```python
from build123d import *

# Parameters (mm, degrees)
SKETCH2_W                = 10
SKETCH2_H                = 10.5
BOSS_EXTRUDE1_DEPTH      = 2
SKETCH3_W                = 12.5
SKETCH3_H                = 14.5
BOSS_EXTRUDE2_DEPTH      = 3.5
SKETCH4_W                = 14.6
SKETCH4_H                = 14.5
BOSS_EXTRUDE3_DEPTH      = 3.5
SKETCH5_W                = 12.5
SKETCH5_H                = 14.5
BOSS_EXTRUDE4_DEPTH      = 4.3
BOSS_EXTRUDE5_DEPTH      = 2.3
SKETCH8_W                = 12.1
SKETCH8_H                = 11.1
CUT_EXTRUDE1_DEPTH       = 13
SKETCH10_W               = 3.5
SKETCH10_H               = 0.7
CUT_EXTRUDE6_DEPTH       = 4
FILLET1_R                = 1
CUT_EXTRUDE9_DEPTH       = 18.994790913
CUT_EXTRUDE9_DEPTH_BACK  = 18.994790913
SKETCH15_W               = 3
SKETCH15_H               = 5
BOSS_EXTRUDE6_DEPTH      = 0.7
FILLET5_R                = 0.5
FILLET3_R                = 1
FILLET4_R                = 1
CUT_EXTRUDE10_DEPTH      = 20.550255917
CUT_EXTRUDE10_DEPTH_BACK = 2
SKETCH14_W               = 4.56
SKETCH14_H               = 10
CHAMFER4_SIZE            = 1.5


with BuildPart() as part:
    # Sketch2 → Boss-Extrude1 (new body)
    with BuildSketch(Plane.YZ):
        Rectangle(SKETCH2_W, SKETCH2_H)
    extrude(amount=BOSS_EXTRUDE1_DEPTH)

    # Sketch3 → Boss-Extrude2 (add)
    with BuildSketch(Plane(origin=(0, 0, 0), x_dir=(0, -1, 0), z_dir=(-1, 0, 0))):
        with Locations((0, 2)):
            Rectangle(SKETCH3_W, SKETCH3_H)
    extrude(amount=BOSS_EXTRUDE2_DEPTH)

    # Sketch4 → Boss-Extrude3 (add)
    with BuildSketch(Plane(origin=(-3.5, 0, 0), x_dir=(0, -1, 0), z_dir=(-1, 0, 0))):
        with Locations((0, 2)):
            Rectangle(SKETCH4_W, SKETCH4_H)
    extrude(amount=BOSS_EXTRUDE3_DEPTH)

    # Sketch5 → Boss-Extrude4 (add)
    with BuildSketch(Plane(origin=(-7, 0, 0), x_dir=(0, -1, 0), z_dir=(-1, 0, 0))):
        with Locations((0, 2)):
            Rectangle(SKETCH5_W, SKETCH5_H)
    extrude(amount=BOSS_EXTRUDE4_DEPTH)

    # Sketch6 → Boss-Extrude5 (add)
    with BuildSketch(Plane(origin=(-11.3, 0, 0), x_dir=(0, -1, 0), z_dir=(-1, 0, 0))):
        Polygon((6.25, -5.25), (7.3, -5.25), (7.3, 9.25), (6.25, 9.25), (-6.25, 9.25), (-7.3, 9.25), (-7.3, -5.25), (-6.25, -5.25), align=None)
    extrude(amount=BOSS_EXTRUDE5_DEPTH)

    # Sketch8 → Cut-Extrude1 (cut)
    with BuildSketch(Plane.XY.offset(9.25)):
        with Locations((-7.55, 0)):
            Rectangle(SKETCH8_W, SKETCH8_H)
    extrude(amount=-CUT_EXTRUDE1_DEPTH, mode=Mode.SUBTRACT)

    # Sketch10 → Cut-Extrude6 (cut)
    with BuildSketch(Plane.XY.offset(9.25)):
        with Locations((-1.75, 5.9)):
            Rectangle(SKETCH10_W, SKETCH10_H)
        with Locations((-1.75, -5.9)):
            Rectangle(SKETCH10_W, SKETCH10_H)
    extrude(amount=-CUT_EXTRUDE6_DEPTH, mode=Mode.SUBTRACT)

    # Fillet1
    fillet1_edges = [part.edges().sort_by_distance(p)[0] for p in [
        (-13.6, -5.55, 2.75),
        (-13.6, 5.55, 2.75),
    ]]
    fillet(fillet1_edges, radius=FILLET1_R)

    # Sketch13 → Cut-Extrude9 (cut, two sides: drawn at the far end of the back side and taken through both)
    with BuildSketch(Plane(origin=(0, 0, 0), x_dir=(0, 0, -1), z_dir=(1, 0, 0)).offset(-CUT_EXTRUDE9_DEPTH_BACK)):
        with BuildLine():
            Line((-2.045, 0.01001), (-2.045, -3.17999))
            ThreePointArc((-2.045, -3.17999), (-1.611518036, -4.226508036), (-0.565, -4.65999))
            Line((-0.565, -4.65999), (0.035, -4.65999))
            ThreePointArc((0.035, -4.65999), (1.081518036, -4.226508036), (1.515, -3.17999))
            Line((1.515, -3.17999), (1.515, 0.01001))
            Line((1.515, 0.01001), (1.515, 3.20001))
            ThreePointArc((1.515, 3.20001), (1.081518036, 4.246528036), (0.035, 4.68001))
            Line((0.035, 4.68001), (-0.565, 4.68001))
            ThreePointArc((-0.565, 4.68001), (-1.611518036, 4.246528036), (-2.045, 3.20001))
            Line((-2.045, 3.20001), (-2.045, 0.01001))
        make_face()
    extrude(amount=CUT_EXTRUDE9_DEPTH + CUT_EXTRUDE9_DEPTH_BACK, mode=Mode.SUBTRACT)

    # Sketch15 → Boss-Extrude6 (add)
    with BuildSketch(Plane.XY.offset(-3.75)):
        with BuildLine():
            Line((-13.6, 6.55), (-13.6, -6.55))
            ThreePointArc((-13.6, -6.55), (-13.307106781, -5.842893219), (-12.6, -5.55))
            Line((-12.6, -5.55), (-1.5, -5.55))
            Line((-1.5, -5.55), (-1.5, 5.55))
            Line((-1.5, 5.55), (-12.6, 5.55))
            ThreePointArc((-12.6, 5.55), (-13.307106781, 5.842893219), (-13.6, 6.55))
        make_face()
        with Locations((-4.5, 0)):
            Rectangle(SKETCH15_W, SKETCH15_H, mode=Mode.SUBTRACT)
    extrude(amount=BOSS_EXTRUDE6_DEPTH)

    # Fillet5
    fillet5_edges = [part.edges().sort_by_distance(p)[0] for p in [
        (-3, 2.5, -3.4),
        (-6, 2.5, -3.4),
        (-6, -2.5, -3.4),
        (-3, -2.5, -3.4),
    ]]
    fillet(fillet5_edges, radius=FILLET5_R)

    # Fillet3
    fillet3_edges = [part.edges().sort_by_distance(p)[0] for p in [
        (-1.5, -5.55, 1.1),
        (-1.5, 5.55, 1.1),
    ]]
    fillet(fillet3_edges, radius=FILLET3_R)

    # Fillet4
    fillet4_edges = [part.edges().sort_by_distance(p)[0] for p in [
        (-13.307106781, 5.842893219, -3.05),
        (-13.307106781, -5.842893219, -3.05),
        (-7.55, -5.55, -3.05),
        (-7.55, 5.55, -3.05),
        (-1.5, 0, -3.05),
        (-1.792893219, -5.257106781, -3.05),
        (-1.792893219, 5.257106781, -3.05),
    ]]
    fillet(fillet4_edges, radius=FILLET4_R)

    # Sketch14 → Cut-Extrude10 (cut, two sides: drawn at the far end of the back side and taken through both)
    with BuildSketch(Plane(origin=(2, 0, 0), x_dir=(0, 0, -1), z_dir=(1, 0, 0)).offset(-CUT_EXTRUDE10_DEPTH_BACK)):
        with Locations((-0.265, 0)):
            Rectangle(SKETCH14_W, SKETCH14_H)
    extrude(amount=CUT_EXTRUDE10_DEPTH + CUT_EXTRUDE10_DEPTH_BACK, mode=Mode.SUBTRACT)

    # Chamfer4
    chamfer4_edges = [part.edges().sort_by_distance(p)[0] for p in [
        (2, 0, 2.545),
        (2, 0, -2.015),
    ]]
    chamfer(chamfer4_edges, length=CHAMFER4_SIZE)


solid = part.part
```
Verification items for the finished model (mm, model axes). A direction names the side the tool comes from. Give positions to 0.01 mm unless a question says otherwise; leave off trailing zeros. Order: outer loops, then holes, each group sorted by start corner. A loop starts at its lowest first (then second) coordinate and runs counter-clockwise, first axis right, second up. Notation, with made-up numbers: M 10.25,42 L 46.25,42 A25 ccw 46.25,66 Z; hole C 4,34 d4. An arc over 180 degrees is marked long. Answer in a Markdown table with one row per item. Add a question column.
Item 1: Section check C-C, the plane y = -1.75. Enter the section's corners in (x, z) (3 decimals).
Item 2: Section check B-B, the plane x = -0.5. Enter the section's corners in (y, z) (3 decimals), and give its area (3 significant figures).
Item 3: Tool access check on faces 4 (the flat face through (-5, 0, -3.75)), 5 (the flat face through (-8, 5.55, 4)), 6 (the flat face through (-9, -6.25, 2)), 7 (the flat face through (-2, -6.25, 0)), 8 (the flat face through (-11.3, 7, 2)). Record the directions out of +Z, -Z, +X, -X, +Y, -Y that give a thin tool (end or side, any length) a straight path to the whole face; none if there is none.
Item 4: Gauge pin test, flat ends, axial feed: pin 1 (1.2 mm diameter, centred on y = -7, z = 0.5, fed in from +X); pin 2 (3 mm diameter, centred on y = 0.5, z = 4, fed in from -X); pin 3 (4 mm diameter, centred on x = -1, z = 0.5, fed in from +Y). Record the tip position at first contact, or that the pin passes through.
Item 5: Mould release check, pull along X, two halves, no side actions. Record for faces 1 (the flat face through (-1, 0, 2.045)), 2 (the flat face through (1.26, 0.07, 3.306)), 3 (the flat face through (-11.3, -7, 2)): released by +X, released by -X, zero draft, split by the parting line, or undercut.
Item 6: Section check A-A, the plane z = 7.25. Enter the section's corners in (x, y).
Item 7: Scan lines: probe 1 along Y at (x, z) = (-11.75, 5); probe 2 along Z at (x, y) = (0.25, -0.5) (3 decimals); probe 3 along X at (y, z) = (-1.5, 8). Record each from-to range of solid material in increasing order. Write a range as from..to.
Item 8: Section check D-D, the plane x = -7.75. Enter the section's corners in (y, z).
Filled sheet:
| question | item | result |
|---|---|---|
| 1 | outline | M -13.6,-5.25 L 2,-5.25 L 2,-3.515 L 0.5,-2.015 L 0,-2.015 L 0,-1.515 L -1.5,-1.515 L -1.5,-2.05 A1 cw -2.5,-3.05 L -3,-3.05 L -3,-3.75 L -6,-3.75 L -6,-3.05 L -13.6,-3.05 Z; M -1.5,2.045 L 0,2.045 L 0,2.545 L 0.5,2.545 L 2,4.045 L 2,5.25 L 0,5.25 L 0,9.25 L -1.5,9.25 Z |
| 2 | outline | M -6.25,-5.25 L 6.25,-5.25 L 6.25,5.25 L 5.55,5.25 L 5.55,9.25 L -5.55,9.25 L -5.55,5.25 L -6.25,5.25 Z; hole M -4.66,-0.035 A1.48 ccw -3.18,-1.515 L 3.2,-1.515 A1.48 ccw 4.68,-0.035 L 4.68,0.565 A1.48 ccw 3.2,2.045 L -3.18,2.045 A1.48 ccw -4.66,0.565 Z |
| 2 | area | 144 mm^2 |
| 3 | face 4 | +Z |
| 3 | face 5 | +Z, -X |
| 3 | face 6 | +Z, -Z, -Y |
| 3 | face 7 | +Z, -Z, +X, -Y |
| 3 | face 8 | +Z, -Z, +Y |
| 4 | pin 1 | stops at x = -3.5 |
| 4 | pin 2 | stops at x = -1.5 |
| 4 | pin 3 | stops at y = 6.25 |
| 5 | face 1 | zero draft |
| 5 | face 2 | released by +X |
| 5 | face 3 | undercut |
| 6 | outline | M -13.6,-7.3 L -11.3,-7.3 L -11.3,-6.25 L -7,-6.25 L -7,-7.3 L -3.5,-7.3 L -3.5,-5.55 L -12.6,-5.55 A1 ccw -13.6,-6.55 Z; M -13.6,6.55 A1 ccw -12.6,5.55 L -3.5,5.55 L -3.5,7.3 L -7,7.3 L -7,6.25 L -11.3,6.25 L -11.3,7.3 L -13.6,7.3 Z; M -1.5,-5.55 L 0,-5.55 L 0,5.55 L -1.5,5.55 Z |
| 7 | probe 1 | y = -7.3..-5.55, 5.55..7.3 |
| 7 | probe 2 | z = -5.25..-2.015, 2.545..5.25 |
| 7 | probe 3 | x = -1.5..0 |
| 8 | outline | M -6.25,-5.25 L 6.25,-5.25 L 6.25,9.25 L 5.55,9.25 L 5.55,-2.05 A1 cw 4.55,-3.05 L -4.55,-3.05 A1 cw -5.55,-2.05 L -5.55,9.25 L -6.25,9.25 Z |
